Source: CAD feature listing. Evaluate the final solid. Frame: model axes, mm. Face numbers are marked on the shaded views. A direction names the side the tool comes from. Give positions to 0.01 mm unless a question says otherwise; leave off trailing zeros. Write each loop counter-clockwise with the first axis right and the second up, starting at its lowest first coordinate (ties: lowest second). Pieces come first, ordered by that corner, then holes. Notation, with made-up numbers: (65, -10.5) -> (83, -10.5) arc R8 cw to (83, -6.5) -> close; hole circle Ø4 at (0, -37.75). An arc over 180 degrees is marked (long way). Write item = value, one per line.
from build123d import *

# Parameters (mm, degrees)
BASPROSKE_W         = 5
BASPROSKE_H         = 11
TOOTHCUT_DEPTH      = 17.340134638
TEETHCUTS_COUNT     = 20
BORSKE_R            = 1.5
BORE_DEPTH          = 50.0000508
SKETCH_1_R          = 6
EXTRUDE_1_DEPTH     = 14
CUT_EXTRUDE_1_DEPTH = 25.468506397
SKETCH_3_R          = 2.7
CUT_EXTRUDE_2_DEPTH = 3


with BuildPart() as part:
    # BasProSke → Base-Revolve (revolve)
    with BuildSketch(Plane(origin=(0, 0, 0), x_dir=(1, 0, 0), z_dir=(0, 1, 0)), mode=Mode.PRIVATE) as base_revolve_sk:
        with Locations((2.5, 5.5)):
            Rectangle(BASPROSKE_W, BASPROSKE_H)
    revolve(base_revolve_sk.sketch.rotate(Axis((-10, 0, 0), (1, 0, 0)), 180), axis=Axis((-10, 0, 0), (1, 0, 0)))

    # TooCutSke → ToothCut (cut, through all)
    with BuildSketch(Plane(origin=(0, 0, 0), x_dir=(0, 0, -1), z_dir=(1, 0, 0))):
        with BuildLine():
            ThreePointArc((0.499924007, 8.734705318), (0, 8.749), (-0.499924007, 8.734705318))
            ThreePointArc((-0.499924007, 8.734705318), (-0.824302243, 9.905497836), (-1.485192705, 10.924909509))
            ThreePointArc((-1.485192705, 10.924909509), (0, 11.0254), (1.485192705, 10.924909509))
            ThreePointArc((1.485192705, 10.924909509), (0.824302243, 9.905497836), (0.499924007, 8.734705318))
        make_face()
    toothcut = extrude(amount=TOOTHCUT_DEPTH, mode=Mode.SUBTRACT)

    # TeethCuts: ToothCut ×20 about axis
    teethcuts_axis = Axis((0, 0, 0), (1, 0, 0))
    for i in range(1, TEETHCUTS_COUNT):
        add(toothcut.rotate(teethcuts_axis, i * 360 / TEETHCUTS_COUNT), mode=Mode.SUBTRACT)

    # BorSke → Bore (cut, symmetric)
    with BuildSketch(Plane(origin=(0, 0, 0), x_dir=(0, 0, -1), z_dir=(1, 0, 0))):
        with Locations(Location((0, 0, 0), (0, 0, 180))):
            Circle(BORSKE_R)
    extrude(amount=BORE_DEPTH, both=True, mode=Mode.SUBTRACT)

    # 草图1 → 凸台-拉伸1 (add)
    with BuildSketch(Plane(origin=(5, 0, 0), x_dir=(0, 0, -1), z_dir=(1, 0, 0))):
        with Locations(Location((0, 0, 0), (0, 0, 180))):
            Circle(SKETCH_1_R)
    extrude(amount=EXTRUDE_1_DEPTH)

    # 草图2 → 切除-拉伸1 (cut, through all)
    with BuildSketch(Plane(origin=(19, 0, 0), x_dir=(0, 0, -1), z_dir=(1, 0, 0))):
        with BuildLine():
            Line((2.2, 1.565247584), (2.2, -1.565247584))
            ThreePointArc((2.2, -1.565247584), (-2.7, 0), (2.2, 1.565247584))
        make_face()
    extrude(amount=-CUT_EXTRUDE_1_DEPTH, mode=Mode.SUBTRACT)

    # 草图3 → 切除-拉伸2 (cut)
    with BuildSketch(Plane(origin=(19, 0, 0), x_dir=(0, 0, -1), z_dir=(1, 0, 0))):
        Circle(SKETCH_3_R)
    extrude(amount=-CUT_EXTRUDE_2_DEPTH, mode=Mode.SUBTRACT)


solid = part.part
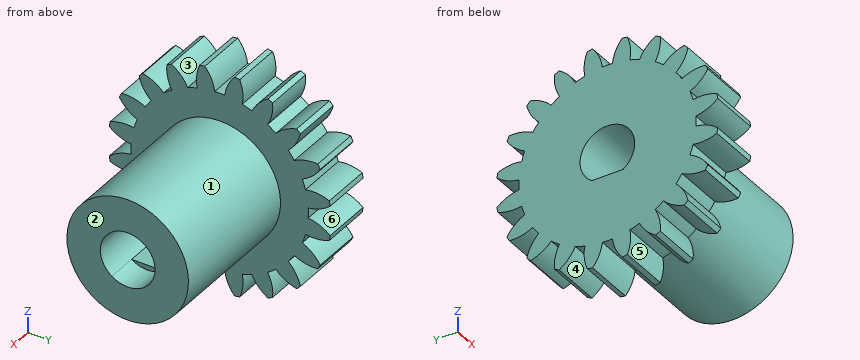
(1) First-contact query: pin 1 (2.5 mm diameter, centred on x = 11, y = -0.5, fed in from +Z); pin 2 (5 mm diameter, centred on x = 14.5, y = -3, fed in from -Z); pin 3 (10 mm diameter, centred on x = 11.5, z = 2, fed in from +Y). Flat tips, straight axial feed; report the tip coordinate or a pass-through.
Values follow:
pin_1 = 6
pin_2 = -5.98
pin_3 = 6
(2) Section query A-A (z = 0). Return loops of the section in (x, y), plus the area to 3 significant figures.
Values follow:
outline = (0, -8.75) -> (5, -8.75) -> (5, -6) -> (19, -6) -> (19, -2.7) -> (0, -2.7) -> close; (0, 2.7) -> (19, 2.7) -> (19, 6) -> (5, 6) -> (5, 8.75) -> (0, 8.75) -> close
area = 153 mm2
(3) Section query B-B (y = 0). Return loops of the section in (x, z), plus the area to 3 significant figures.
Values follow:
outline = (0, -8.75) -> (5, -8.75) -> (5, -6) -> (19, -6) -> (19, -2.7) -> (16, -2.7) -> (16, -2.2) -> (0, -2.2) -> close; (0, 2.7) -> (19, 2.7) -> (19, 6) -> (5, 6) -> (5, 8.75) -> (0, 8.75) -> close
area = 161 mm2
(4) Material intervals for line 1 (Y direction, x = 11.75, z = 0); line 2 (X direction, y = -2.5, z = 7.25); line 3 (Y direction, x = 3.75, z = 7.5), sorted ascending.
Values follow:
line_1 = -6 to -2.7, 2.7 to 6
line_2 = 0 to 5
line_3 = -7.94 to -6.44, -4.8 to 4.8, 6.44 to 7.94
(5) Pull-direction query (Y, two-part tool) for the marked faces 1, 2 and 3; classes: pulls with the +Y half, pulls with the -Y half, needs draft (parallel to the pull), parting line crosses it, or undercut.
Values follow:
face_1 = parting line crosses it
face_2 = needs draft
face_3 = undercut
(6) Access query for the marked faces 4, 5 and 6. Directions: +Z, -Z, +X, -X, +Y, -Y. A direction counts if a zero-diameter tool reaches every point of the face in a straight line with its end or side. Return the directions, or none.
Values follow:
face_4 = -Z, +X, -X
face_5 = +X, -X
face_6 = +X, -X, +Y
(7) Section query D-D (x = 12). Return loops of the section in (y, z), plus the area to 3 significant figures.
Values follow:
outline = circle Ø12 at (0, 0); hole (-1.57, -2.2) -> (1.57, -2.2) arc R2.7 ccw (long way) to start
area = 91.3 mm2
(8) Section query C-C (z = -9.25). Return loops of the section in (x, y).
Values follow:
outline = (0, -5.24) -> (5, -5.24) -> (5, -3.92) -> (0, -3.92) -> close; (0, -2.3) -> (5, -2.3) -> (5, -0.6) -> (0, -0.6) -> close; (0, 0.6) -> (5, 0.6) -> (5, 2.3) -> (0, 2.3) -> close; (0, 3.92) -> (5, 3.92) -> (5, 5.24) -> (0, 5.24) -> close
